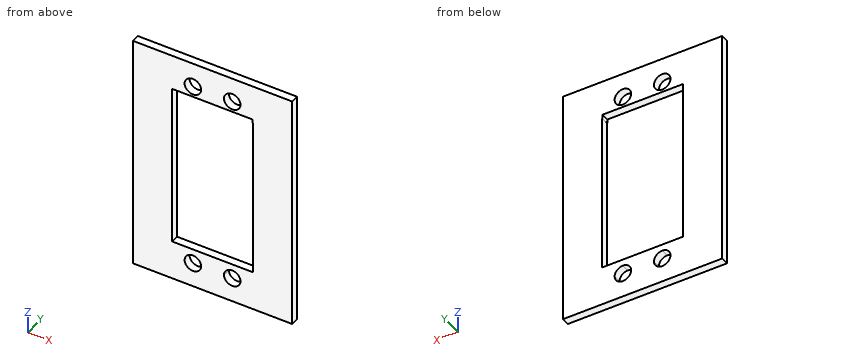
```python
from build123d import *

# Parameters (mm, degrees)
SKETCH_1_W          = 40.5
SKETCH_1_H          = 60.5
SKETCH_1_R          = 2.1
EXTRUDE_2_DEPTH     = 2
SKETCH_3_W          = 20.471244586
SKETCH_3_H          = 1
CUT_EXTRUDE_2_DEPTH = 2


with BuildPart() as part:
    # 草图1 → 凸台-拉伸2 (new body)
    # profile 1 of 2: a face of its own
    with BuildSketch(Plane(origin=(0, 0, 0), x_dir=(1, 0, 0), z_dir=(0, 1, 0))):
        Rectangle(SKETCH_1_W, SKETCH_1_H)
        with Locations(Location((-5, -24, 0), (0, 0, 270))):
            Circle(SKETCH_1_R, mode=Mode.SUBTRACT)
        with Locations(Location((5, -24, 0), (0, 0, 270))):
            Circle(SKETCH_1_R, mode=Mode.SUBTRACT)
        with BuildLine():
            Line((10.25, -20.25), (-10.25, -20.25))
            Line((-10.25, -20.25), (-10.25, 20.25))
            Line((-10.25, 20.25), (-5, 20.25))
            Line((-5, 20.25), (-5, 21.9))
            ThreePointArc((-5, 21.9), (-6.48492424, 25.48492424), (-2.9, 24))
            Line((-2.9, 24), (2.9, 24))
            ThreePointArc((2.9, 24), (5, 26.1), (7.1, 24))
            ThreePointArc((7.1, 24), (6.48492424, 22.51507576), (5, 21.9))
            Line((5, 21.9), (5, 20.25))
            Line((5, 20.25), (10.25, 20.25))
            Line((10.25, 20.25), (10.25, -20.25))
        make_face(mode=Mode.SUBTRACT)
    # profile 2 of 2: a face of its own
    with BuildSketch(Plane(origin=(0, 0, 0), x_dir=(1, 0, 0), z_dir=(0, 1, 0))):
        with BuildLine():
            Line((-5, 21.9), (-5, 20.25))
            Line((-5, 20.25), (5, 20.25))
            Line((5, 20.25), (5, 21.9))
            ThreePointArc((5, 21.9), (3.51507576, 22.51507576), (2.9, 24))
            Line((2.9, 24), (-2.9, 24))
            ThreePointArc((-2.9, 24), (-3.51507576, 22.51507576), (-5, 21.9))
        make_face()
    extrude(amount=EXTRUDE_2_DEPTH)

    # 草图3 → 切除-拉伸2 (cut)
    with BuildSketch(Plane(origin=(0, 2, 0), x_dir=(1, 0, 0), z_dir=(0, 1, 0))):
        with Locations((-0.014377707, -20.75)):
            Rectangle(SKETCH_3_W, SKETCH_3_H)
    extrude(amount=-CUT_EXTRUDE_2_DEPTH, mode=Mode.SUBTRACT)


solid = part.part
```
Geometry: final body of the model. Coordinates: model frame, mm. Round coordinates to 2 decimals unless told otherwise and drop trailing zeros. Order: outer loops, then holes, each group sorted by start corner. A loop starts at its lowest first (then second) coordinate and runs counter-clockwise, first axis right, second up. Notation, with made-up numbers: (-17.5, 35.5) -> (22.5, 35.5) arc R24 ccw to (22.5, 45.5) -> close; hole circle Ø6 at (49.25, -2.75). An arc over 180 degrees is marked (long way). Use one line per item in the form item = value. Start each with the question number.
1. Pin query (flat end, axial travel): pin 1 Ø4 at (x, z) = (5, 24) entering from -Y. Return the tip coordinate at first contact, or that it passes through.
2. Cut plane D-D (y = 1.6). Count the separate pieces of the cut face and the enclosed holes in it, then the cut area to 3 significant figures.
3. Cut plane A-A (x = 9). Return the cut outline in (y, z).
4. Line query: probe 1 along X at (y, z) = (0.8, 24); probe 2 along X at (y, z) = (0.3, 2); probe 3 along Z at (x, y) = (2, 1.1). Output: solid intervals per line, ascending.
5. Cut plane B-B (z = 11). Return the cut outline in (x, y), then the cut area to 3 significant figures.
6. Cut plane C-C (z = 24). Return the cut outline in (x, y), then the cut area to 3 significant figures.
Solution:
q1.pin_1 = through
q2.separate_pieces = 1
q2.enclosed_holes = 5
q2.area = 1,540 mm^2
q3.outline = (0, -30.25) -> (2, -30.25) -> (2, -20.25) -> (0, -20.25) -> close; (0, 21.25) -> (2, 21.25) -> (2, 30.25) -> (0, 30.25) -> close
q4.probe_1 = -20.25 to -7.1, -2.9 to 2.9, 7.1 to 20.25
q4.probe_2 = -20.25 to -10.25, 10.25 to 20.25
q4.probe_3 = -30.25 to -20.25, 21.25 to 30.25
q5.outline = (-20.25, 0) -> (-10.25, 0) -> (-10.25, 2) -> (-20.25, 2) -> close; (10.25, 0) -> (20.25, 0) -> (20.25, 2) -> (10.25, 2) -> close
q5.area = 40.0 mm^2
q6.outline = (-20.25, 0) -> (-7.1, 0) -> (-7.1, 2) -> (-20.25, 2) -> close; (-2.9, 0) -> (2.9, 0) -> (2.9, 2) -> (-2.9, 2) -> close; (7.1, 0) -> (20.25, 0) -> (20.25, 2) -> (7.1, 2) -> close
q6.area = 64.2 mm^2
